Geometry: final body of the model. Coordinates: model frame, mm. A direction names the side the tool comes from. Give positions to 0.01 mm unless a question says otherwise; leave off trailing zeros. Order: outer loops, then holes, each group sorted by start corner. A loop starts at its lowest first (then second) coordinate and runs counter-clockwise, first axis right, second up. Notation, with made-up numbers: (-19, 36) - (-4, 36) arc R16 ccw to (-4, 66) - close; hole circle Ø6 at (-33.75, 30). An arc over 180 degrees is marked (long way). One line per item, written item: value.
Autodesk Inventor part; units mm, degrees
ref_plane "YZ Plane" through (0, 0, 0) normal (1, 0, 0) x (0, 1, 0)
ref_plane "XZ Plane" through (0, 0, 0) normal (0, 1, 0) x (-1, 0, 0)
ref_plane "XY Plane" through (0, 0, 0) normal (0, 0, 1) x (1, 0, 0)
sketch "Sketch1" plane through (0, 0, 0) normal (1, 0, 0) x (0, 1, 0)
  circle A0 centre (-2.6054, -169.98) radius 2.05
  arc A1 (17.5, -0.0099) -> (-16.9792, -4.2375) centre (0, 0) ccw
  arc A2 (-7.5969, -170.2704) -> (1.9242, -172.0973) centre (-2.6054, -169.98) ccw
  line L0 (17.5, -0.0099) -> (47.8897, -0.0099) construction
  line L1 (17.5, -0.0099) -> (24.6336, -122.6611)
  line L2 (24.3565, -124.1056) -> (1.9242, -172.0973)
  line L3 (-17.5, -0.0032) -> (-2.3777, -122.9531)
  line L4 (-2.3898, -123.7729) -> (-8.122, -161.2434)
  line L5 (-17.5, -0.0032) -> (-17.3824, -2.0256)
  line L6 (-8.122, -161.2434) -> (-7.5969, -170.2704)
  arc A3 (24.3565, -124.1056) -> (24.6336, -122.6611) centre (21.6387, -122.8353) ccw
  arc A4 (-2.3898, -123.7729) -> (-2.3777, -122.9531) centre (-5.3553, -123.3193) ccw
  circle A5 centre (4.5959, -51.0056) radius 9
  circle A6 centre (11.1072, -123.2673) radius 6
  circle A7 centre (0, 0) radius 12.5
  line L7 (12.5, 0) -> (17.103, -123.043)
  line L8 (-12.5, 0) -> (5.1072, -123.2673)
  point P0 (-2.3556, -123.3634)
  point P1 (24.5849, -123.4006)
  point P2 (-12.0001, -3.4995)
  dimension "d8" = 10
  dimension "d9" = 35
  dimension "d10" = 4.1
  dimension "d11" = 170
  dimension "d12" = 3
  dimension "d13" = 3
  dimension "d16" = 18
  dimension "d17" = 12
  dimension "d19" = 25
extrude "Extrusion1" add sketch "Sketch1" along normal blind 4 contours L1 A3 L2 A2 L6 L4 A4 L3 A1
extrude "Extrusion2" add sketch "Sketch1" along normal blind 3 contours A6 L8 A7 L7
extrude "Extrusion3" add sketch "Sketch1" along normal blind 3 contours A7 L8 picked at (2.216, 2.7519)
equation "\"BendRadius\" = Thickness"
equation "\"BendReliefWidth\" = Thickness"
equation "\"BendReliefDepth\" = 0.5 * Thickness"
equation "\"CornerReliefSize\" = 4 * Thickness"
equation "\"MinimumRemnant\" = 2 * Thickness"
equation "\"TransitionRadius\" = BendRadius"
equation "\"JacobiRadiusSize\" = BendRadius"
equation "\"GapSize\" = Thickness"
properties part number "LINK1"
1) Section C-C, the plane z = -95. Return loops of the section in (x, y), then the cut area to 3 significant figures.
Answers below:
outline: (0, -5.82) - (4, -5.82) - (4, 1.07) - (3, 1.07) - (3, 16.05) - (4, 16.05) - (4, 23.02) - (0, 23.02) - close
area: 100 mm^2
2) Material intervals for line 1 along Z through (x, y) = (2.3, 12.5); line 2 along Z through (x, y) = (1.75, 5); line 3 along X through (y, z) = (12, -25), sorted ascending.
Answers below:
line 1: -149.47 to -129.1, -117.43 to -55.31, -46.7 to 12.25
line 2: -165.52 to -60, -42.01 to 16.77
line 3: 0 to 3
3) Section A-A, the plane x = 1.7. Return loops of the section in (y, z), then the cut area to 3 significant figures.
Answers below:
outline: (-17.5, 0) - (-2.38, -122.95) arc R3 cw to (-2.39, -123.77) - (-8.12, -161.24) - (-7.6, -170.27) arc R5 ccw to (1.92, -172.1) - (24.36, -124.11) arc R3 ccw to (24.63, -122.66) - (17.5, -0.01) arc R17.5 ccw to start; hole (-12.5, 0) arc R12.5 ccw to (-12, -3.5) - close; hole circle Ø4.1 at (-2.61, -169.98); hole circle Ø18 at (4.6, -51.01); hole circle Ø12 at (11.11, -123.27)
area: 4,870 mm^2
4) Set-up query: faces 1 (the face through (1.972, -7.863, -165.694)), 2 (the face through (1.972, -10.045, -60.618)), 3 (the face through (3.49, 14.77, -60.66)). Return all of +Z, -Z, +X, -X, +Y, -Y with unobstructed straight access to the full face (end or side cutting, diameter ignored); none if empty.
Answers below:
face 1: -Z, +X, -X, -Y
face 2: +X, -X, -Y
face 3: +X
5) Section D-D, the plane z = -64.5. Return loops of the section in (x, y), then the cut area to 3 significant figures.
Answers below:
outline: (0, -9.57) - (4, -9.57) - (4, -3.29) - (3, -3.29) - (3, 14.91) - (4, 14.91) - (4, 21.25) - (0, 21.25) - close
area: 105 mm^2
6) Section B-B, the plane y = 7. Return loops of the section in (x, z), then the cut area to 3 significant figures.
Answers below:
outline: (0, -161.24) - (4, -161.24) - (4, -127.64) - (0, -127.64) - close; (0, -118.89) - (3, -118.89) - (3, -59.68) - (0, -59.68) - close; (0, -42.33) - (3, -42.33) - (3, 10.36) - (4, 10.36) - (4, 16.04) - (0, 16.04) - close
area: 493 mm^2
7) Mould query, pull axis Z, two halves, no side actions, for faces 4 (the face through (1.972, 13.297, -147.766)), 5 (the face through (3.493, -3.566, -62.545)), 6 (the face through (0, 13, -56)), 7 (the face through (1.97, -3.05, -167.98)). Classes: released by +Z, released by -Z, zero draft, split by the parting line, or undercut.
Answers below:
face 4: released by -Z
face 5: undercut
face 6: zero draft
face 7: undercut
8) First-contact query: pin 1 (5 mm diameter, centred on y = 17.5, z = -142, fed in from +X); pin 2 (2 mm diameter, centred on x = 3, y = 14, fed in from -Z); pin 3 (1 mm diameter, centred on x = 2.5, z = -122.5, fed in from -Y). Flat tips, straight axial feed; report the tip coordinate or a pass-through.
Answers below:
pin 1: x = 4
pin 2: z = -148.4
pin 3: y = -2.49
